from build123d import *

# Parameters (mm, degrees)
F0_R     = 7
F1_DEPTH = 43


with BuildPart() as f1:
    # F0 (on Front) → F1 (new body)
    with BuildSketch(Plane.XZ):
        with BuildLine():
            Line((0, 18), (0, 0))
            Line((0, 0), (7, -7))
            Line((7, -7), (14, -7))
            Line((14, -7), (35.066626, -7))
            ThreePointArc((35.066626, -7), (38.331862, -8.213414), (40.012265, -11.264706))
            ThreePointArc((40.012265, -11.264706), (42.349095, -19.115672), (46.788067, -26))
            Line((46.788067, -26), (52, -26))
            Line((52, -26), (81, 7))
            Line((81, 7), (81, 26))
            Line((81, 26), (76, 31))
            Line((76, 31), (56.832022, 31))
            ThreePointArc((56.832022, 31), (48.381545, 22.690776), (36.650578, 21.006092))
            Line((36.650578, 21.006092), (14, 25))
            Line((14, 25), (7, 25))
            Line((7, 25), (0, 18))
        make_face()
        with Locations((14, 7)):
            Circle(F0_R, mode=Mode.SUBTRACT)
    extrude(amount=F1_DEPTH)


solid = f1.part
Geometry: final body of the model. Coordinates: model frame, mm. A direction names the side the tool comes from. Round coordinates to 2 decimals unless told otherwise and drop trailing zeros. Order: outer loops, then holes, each group sorted by start corner. A loop starts at its lowest first (then second) coordinate and runs counter-clockwise, first axis right, second up. Notation, with made-up numbers: (-22, 77.25) -> (37, 77.25) arc R19 ccw to (37, 105.25) -> close; hole circle Ø6 at (-10, -11.5). An arc over 180 degrees is marked (long way). Put each result on its own line as item: value. Start each with the question number.
Q1. Pull-direction query (X, two-part tool) for faces 4 (the flat face through (81, -21, 16)), 5 (the flat face through (40, 0, 9)), 6 (the flat face through (25.484, -21.199, 22.975)), 7 (the flat face through (4, -21, 22)); classes: +X half, -X half, draft (parallel to the pull), parting line (faces both ways), or undercut.
Q2. First-contact query: pin 1 (4 mm diameter, centred on y = -17.5, z = -19, fed in from +X); pin 2 (8.5 mm diameter, centred on x = 22, y = -27.5, fed in from -Z); pin 3 (3 mm diameter, centred on x = 50.5, y = -25, fed in from +Z). Flat tips, straight axial feed; report the tip coordinate or a pass-through.
Q3. Reachability of faces 1 (the flat face through (11, -21, 25)), 2 (the flat face through (67, -21, 31)), 3 (the flat face through (21, -21, -7)) from +Z, -Z, +X, -X, +Y, -Y: full face, straight path, thin tool, end or side. Return the list, or none.
Q4. Section A-A on x = 16.5. Return the cut outline in (y, z).
Q5. Section D-D on z = 19.5. Return the cut outline in (x, y).
Q6. Section C-C on y = -13. Return the cut outline in (x, z).
Q7. Section B-B on z = 12. Return the cut outline in (x, y).
Q8. Line query: probe 1 along Z at (x, y) = (14, -13); probe 2 along X at (y, z) = (-28, 11); probe 3 along X at (y, z) = (-36, 1.5). Output: solid intervals per line, ascending.
Ans:
1. face 4: +X half
1. face 5: draft
1. face 6: undercut
1. face 7: -X half
2. pin 1: stops at x = 59.91
2. pin 2: stops at z = -7
2. pin 3: stops at z = 25.03
3. face 1: +Z, -X, +Y, -Y
3. face 2: +Z, +X, -X, +Y, -Y
3. face 3: -Z, -X, +Y, -Y
4. outline: (-43, -7) -> (0, -7) -> (0, 0.46) -> (-43, 0.46) -> close; (-43, 13.54) -> (0, 13.54) -> (0, 24.56) -> (-43, 24.56) -> close
5. outline: (1.5, -43) -> (81, -43) -> (81, 0) -> (1.5, 0) -> close
6. outline: (0, 0) -> (7, -7) -> (35.07, -7) arc R5 cw to (40.01, -11.26) arc R29 ccw to (46.79, -26) -> (52, -26) -> (81, 7) -> (81, 26) -> (76, 31) -> (56.83, 31) arc R19 cw to (36.65, 21.01) -> (14, 25) -> (7, 25) -> (0, 18) -> close; hole circle Ø14 at (14, 7)
7. outline: (0, -43) -> (9.1, -43) -> (9.1, 0) -> (0, 0) -> close; (18.9, -43) -> (81, -43) -> (81, 0) -> (18.9, 0) -> close
8. probe 1: z = -7 to 0, 14 to 25
8. probe 2: x = 0 to 8.26, 19.74 to 81
8. probe 3: x = 0 to 9.67, 18.33 to 76.17
